Could you check a few things on this model? Use its own coordinates, in mm. Face numbers are marked on the shaded views. A direction names the side the tool comes from. Coordinates: 2 decimals unless noted, no trailing zeros. Loops run counter-clockwise (first coordinate to the right, second up) from the corner with the lowest first, then second, coordinate; pieces in that order, holes last. Notation, with made-up numbers: (-2.75, 85.5) -> (34.25, 85.5) arc R20 ccw to (34.25, 118.5) -> close; hole circle Ø4 at (-36, -29.5). An arc over 180 degrees is marked (long way). One line per question, with ' | ' between items.
```python
from build123d import *

# Parameters (mm, degrees)
PAD_DEPTH    = 20
SKETCH001_W  = 30
SKETCH001_H  = 50
PAD001_DEPTH = 20
SKETCH004_R  = 4
POCKET_DEPTH = 5


with BuildPart() as part:
    # Sketch → Pad (new body)
    with BuildSketch(Plane.XY):
        Polygon((0, 0), (0, 50), (60, 50), (100, 20), (100, 0), align=None)
    extrude(amount=PAD_DEPTH)

    # Sketch001 (on Face7 of Pad) → Pad001 (join)
    with BuildSketch(Plane.XY.offset(20)):
        with Locations((15, 25)):
            Rectangle(SKETCH001_W, SKETCH001_H)
    extrude(amount=PAD001_DEPTH)

    # Sketch004 (on Face7 of Pad001) → Pocket (cut)
    with BuildSketch(Plane(origin=(0, 0, 0), x_dir=(0, -1, 0), z_dir=(-1, 0, 0))):
        with Locations((-10, 10)):
            Circle(SKETCH004_R)
    extrude(amount=-POCKET_DEPTH, mode=Mode.SUBTRACT)


solid = part.part
```
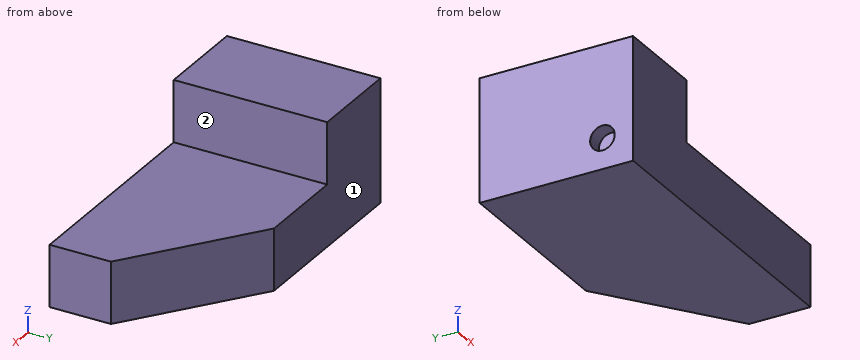
Q1. For pin 1 (25 mm diameter, centred on x = 60.5, y = 35, fed in from +Z); pin 2 (4 mm diameter, centred on y = 9.5, z = 10, fed in from -X); pin 3 (22 mm diameter, centred on y = 31, z = 32.5, fed in from +X), each with a flat end and sliding along its axis, tell me the tip position at first contact or that it passes through.
Values follow:
pin 1: stops at z = 20 | pin 2: stops at x = 5 | pin 3: stops at x = 30
Q2. For the marked faces 1 and 2, which set-ups out of +Z, -Z, +X, -X, +Y, -Y let a thin tool reach every point of the face, with its end or its side?
Values follow:
face 1: +Z, -Z, +X, -X, +Y | face 2: +Z, +X, +Y, -Y
Q3. Imagine slicing it at A-A on z = 10. Write out the boundary of the cut face in (x, y).
Values follow:
outline: (0, 0) -> (100, 0) -> (100, 20) -> (60, 50) -> (0, 50) -> (0, 14) -> (5, 14) -> (5, 6) -> (0, 6) -> close
Q4. Imagine slicing it at B-B on y = 10. Write out the boundary of the cut face in (x, z), plus the area to 3 significant figures.
Values follow:
outline: (0, 0) -> (100, 0) -> (100, 20) -> (30, 20) -> (30, 40) -> (0, 40) -> (0, 14) -> (5, 14) -> (5, 6) -> (0, 6) -> close | area: 2,560 mm2
Q5. Please list where these lines run through material, in increasing order: L1, parallel to Z at x = 1, y = 10; L2, parallel to X at y = 35.5, z = 29.5; L3, parallel to Z at x = 35, y = 29. Write a range as [from, to].
Values follow:
L1: z = [0, 6], [14, 40] | L2: x = [0, 30] | L3: z = [0, 20]
Q6. Imagine slicing it at C-C on x = 81. Write out the boundary of the cut face in (y, z).
Values follow:
outline: (0, 0) -> (34.25, 0) -> (34.25, 20) -> (0, 20) -> close
Q7. Imagine slicing it at D-D on y = 3.5. Write out the boundary of the cut face in (x, z), plus the area to 3 significant figures.
Values follow:
outline: (0, 0) -> (100, 0) -> (100, 20) -> (30, 20) -> (30, 40) -> (0, 40) -> close | area: 2,600 mm2
